Geometry check sheet. Reference: drawing and pictorial views, mm from the part's lowest x, y, z. A direction names the side the tool comes from. Coordinates: 2 decimals unless noted, no trailing zeros. Write each loop counter-clockwise with the first axis right and the second up, starting at its lowest first coordinate (ties: lowest second). Pieces come first, ordered by that corner, then holes. Notation, with made-up numbers: (48, 81) -> (90, 81) arc R12 ccw to (90, 85) -> close; hole circle Ø2 at (-35.5, 62). An arc over 180 degrees is marked (long way). Answer in a Markdown table with one row per item.
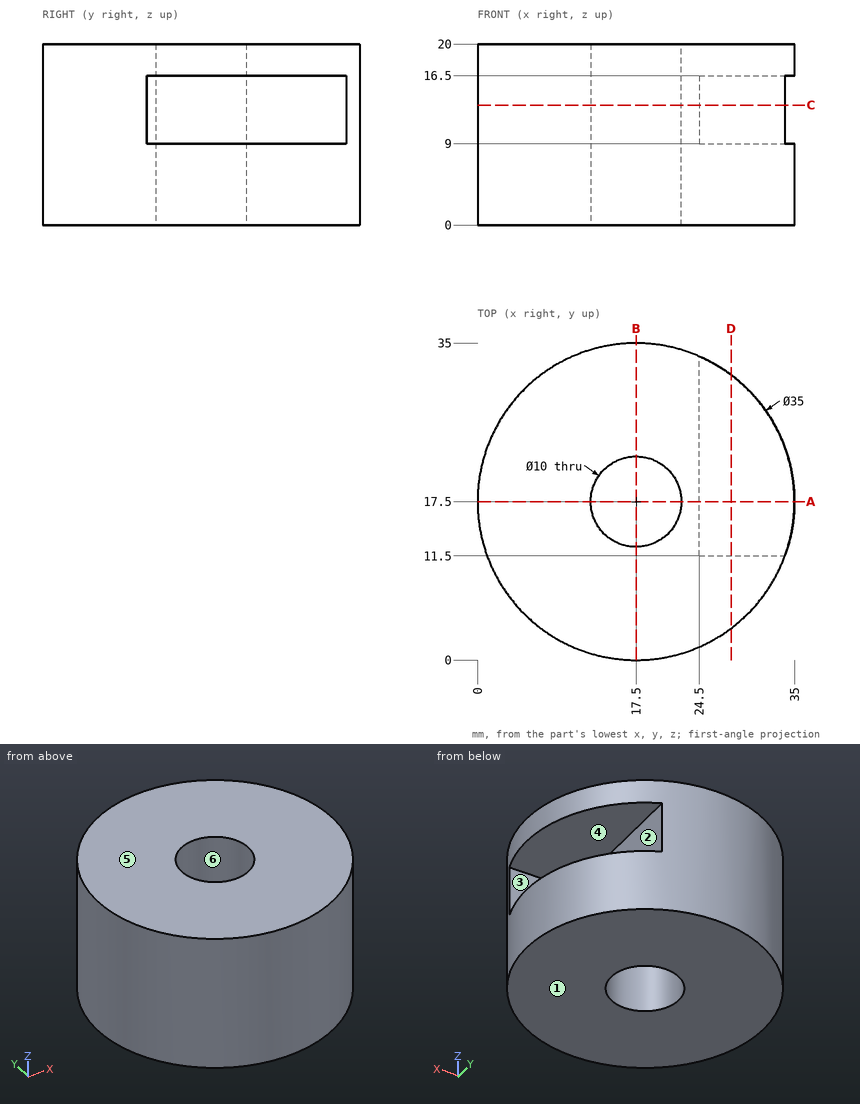
1. Section check A-A, the plane y = 17.5. Record the boundary of the cut face in (x, z).
Geometry says:
| item | result |
|---|---|
| outline | (0, 0) -> (12.5, 0) -> (12.5, 20) -> (0, 20) -> close; (22.5, 0) -> (35, 0) -> (35, 9) -> (24.5, 9) -> (24.5, 16.5) -> (35, 16.5) -> (35, 20) -> (22.5, 20) -> close |
2. Section check C-C, the plane z = 13.25. Record the boundary of the cut face in (x, y), plus the area to 3 significant figures.
Geometry says:
| item | result |
|---|---|
| outline | (24.5, 11.5) -> (24.5, 33.54) arc R17.5 ccw (long way) to (33.94, 11.5) -> close; hole circle Ø10 at (17.5, 17.5) |
| area | 701 mm^2 |
3. Depth check by flat-ended pin: P1, Ø1, axis at y = 8, z = 9, coming from the -X side; P2, Ø13, axis at x = 17.5, y = 17.5, coming from the +Z side; P3, Ø6, axis at x = 31, z = 13, coming from the +Y side; P4, Ø2, axis at x = 14.5, z = 5.5, coming from the +Y side. Enter the tip coordinate at first touch or a pass-through.
Geometry says:
| item | result |
|---|---|
| P1 | x = 2.49 |
| P2 | z = 20 |
| P3 | y = 11.5 |
| P4 | y = 34.89 |
4. Tool access check on the marked faces 1 and 2. Record the directions out of +Z, -Z, +X, -X, +Y, -Y that give a thin tool (end or side, any length) a straight path to the whole face; none if there is none.
Geometry says:
| item | result |
|---|---|
| face 1 | -Z, +X, -X, +Y, -Y |
| face 2 | +X, +Y |
5. Mould release check, pull along Z, two halves, no side actions. Record for the marked faces 3, 4, 5 and 6: released by +Z, released by -Z, zero draft, split by the parting line, or undercut.
Geometry says:
| item | result |
|---|---|
| face 3 | undercut |
| face 4 | undercut |
| face 5 | released by +Z |
| face 6 | zero draft |
6. Section check B-B, the plane x = 17.5. Record the boundary of the cut face in (y, z), plus the area to 3 significant figures.
Geometry says:
| item | result |
|---|---|
| outline | (0, 0) -> (12.5, 0) -> (12.5, 20) -> (0, 20) -> close; (22.5, 0) -> (35, 0) -> (35, 20) -> (22.5, 20) -> close |
| area | 500 mm^2 |
7. Thickness scan on line 1 (Y direction, x = 17.5, z = 13.75); line 2 (Z direction, x = 31.5, y = 18.5); line 3 (X direction, y = 15, z = 18). Record the ranges inside material, lowest first. Write a range as from..to.
Geometry says:
| item | result |
|---|---|
| line 1 | 0..12.5, 22.5..35 |
| line 2 | 0..9, 16.5..20 |
| line 3 | 0.18..13.17, 21.83..34.82 |
8. Section check D-D, the plane x = 28. Record the boundary of the cut face in (y, z).
Geometry says:
| item | result |
|---|---|
| outline | (3.5, 0) -> (31.5, 0) -> (31.5, 9) -> (11.5, 9) -> (11.5, 16.5) -> (31.5, 16.5) -> (31.5, 20) -> (3.5, 20) -> close |
